For this review, take the finished solid that the model builds, in its own axes (mm). Coordinates: 2 decimals unless noted, no trailing zeros. Write each loop counter-clockwise with the first axis right and the second up, starting at its lowest first coordinate (ties: lowest second). Pieces come first, ordered by that corner, then holes. Notation, with made-up numbers: (-3.5, 55) -> (33.5, 55) arc R9 ccw to (33.5, 66) -> close; hole circle Ø2 at (-8, 22). An arc over 180 degrees is marked (long way). Put each result on its own line as item: value. Start each with the question number.
Item 1: To check wall thickness, follow L1, parallel to X at y = 69.85, z = 4 (3 decimals); L2, parallel to X at y = 59.5, z = 1.5; L3, parallel to X at y = 46, z = 6.25. State the ranges of each line that lie inside material, in increasing order.
Item 2: Consider section B-B on y = 25.4. Give the boundary of the cut face in (x, z), and give its area (3 significant figures).
Item 3: Consider section C-C on z = 1. Give the boundary of the cut face in (x, y) (3 decimals), and give its area (3 significant figures).
Item 4: Consider section A-A on x = 247.65. Give the boundary of the cut face in (y, z), and give its area (3 significant figures).
Item 5: Consider section D-D on y = 50.8. Give the boundary of the cut face in (x, z).
Autodesk Inventor part; units mm, degrees
ref_plane "YZ Plane" through (0, 0, 0) normal (1, 0, 0) x (0, 1, 0)
ref_plane "XZ Plane" through (0, 0, 0) normal (0, 1, 0) x (-1, 0, 0)
ref_plane "XY Plane" through (0, 0, 0) normal (0, 0, 1) x (1, 0, 0)
sketch "Sketch1" plane through (0, 0, 0) normal (0, 0, 1) x (1, 0, 0)
  line L0 (0, 0) -> (444.5, 0)
  line L1 (444.5, 0) -> (444.5, 76.2)
  line L2 (444.5, 76.2) -> (0, 76.2)
  line L3 (0, 76.2) -> (0, 0)
  dimension "d0" = 444.5
  dimension "d1" = 76.2
extrude "Extrusion1" add sketch "Sketch1" along normal blind 6.35
chamfer "Chamfer1" distance 12.7 angle 45 1 edges at (444.5, 0, 3.175)
chamfer "Chamfer2" distance 12.7 angle 45 1 edges at (0, 0, 3.175)
sketch "Sketch2" plane through (0, 0, 6.35) normal (0, 0, 1) x (1, 0, 0)
  line L0 (0, 46.8514) -> (152.4, 46.8514)
  line L1 (444.5, 12.7) -> (444.5, 76.2)
  line L2 (292.1, 46.8514) -> (444.5, 46.8514)
  circle A0 centre (152.4, 46.8514) radius 12.7
  circle A1 centre (292.1, 46.8514) radius 12.7
  point P0 (0, 0)
  point P1 (139.7, 46.8514)
  point P2 (165.1, 46.8514)
  dimension "d10" = 152.4
  dimension "d11" = 25.4
  dimension "d12" = 25.4
extrude "Extrusion2" cut sketch "Sketch2" against normal blind 25.4
sketch "Sketch3" plane through (0, 0, 6.35) normal (0, 0, 1) x (1, 0, 0)
  circle A0 centre (152.4, 46.8514) radius 12.7
  line L0 (139.7, 46.8514) -> (139.7, 76.2)
  line L1 (165.1, 46.8514) -> (165.1, 76.2)
  line L2 (444.5, 76.2) -> (0, 76.2)
  line L3 (139.7, 76.2) -> (165.1, 76.2)
  arc A1 (139.7, 46.8514) -> (165.1, 46.8514) centre (152.4, 46.8514) ccw
  point P0 (0, 0)
extrude "Extrusion3" cut sketch "Sketch3" against normal blind 25.4 contours A0 L0 L2 L1
sketch "Sketch4" plane through (0, 0, 6.35) normal (0, 0, 1) x (1, 0, 0)
  circle A0 centre (292.1, 46.8514) radius 12.7
  line L0 (279.4, 46.8514) -> (279.4, 76.2)
  line L1 (444.5, 76.2) -> (165.1, 76.2)
  line L2 (304.8, 46.8514) -> (304.8, 76.2)
  line L3 (304.8, 76.2) -> (279.4, 76.2)
  arc A1 (279.4, 46.8514) -> (304.8, 46.8514) centre (292.1, 46.8514) ccw
  point P0 (0, 0)
extrude "Extrusion4" cut sketch "Sketch4" against normal blind 25.4 contours A0 L0 L1 L2
sketch "Sketch5" plane through (0, 0, 6.35) normal (0, 0, 1) x (1, 0, 0)
  line L0 (0, 76.2) -> (0, 12.7)
  line L1 (12.7, 0) -> (431.8, 0)
  line L2 (444.5, 12.7) -> (444.5, 76.2)
  circle A0 centre (50.8, 25.4) radius 6.35
  circle A1 centre (393.7, 25.4) radius 6.35
  point P0 (0, 0)
  dimension "d19" = 50.8
  dimension "d20" = 25.4
  dimension "d21" = 25.4
  dimension "d22" = 50.8
  dimension "d23" = 12.7
  dimension "d24" = 12.7
extrude "Extrusion5" cut sketch "Sketch5" against normal blind 25.4
sketch "Sketch6" plane through (0, 0, 6.35) normal (0, 0, 1) x (1, 0, 0)
  line L0 (139.7, 76.2) -> (0, 76.2)
  line L1 (0, 76.2) -> (0, 12.7)
  line L2 (444.5, 76.2) -> (304.8, 76.2)
  line L3 (444.5, 12.7) -> (444.5, 76.2)
  circle A0 centre (6.35, 69.85) radius 0.635
  circle A1 centre (438.15, 69.85) radius 0.635
  point P0 (0, 0)
  dimension "d27" = 6.35
  dimension "d28" = 6.35
  dimension "d29" = 6.35
  dimension "d30" = 6.35
  dimension "d31" = 1.27
  dimension "d32" = 1.27
extrude "Extrusion6" cut sketch "Sketch6" against normal blind 25.4
sketch "Sketch7" plane through (0, 0, 6.35) normal (0, 0, 1) x (1, 0, 0)
  line L0 (279.4, 76.2) -> (165.1, 76.2)
  line L1 (165.1, 76.2) -> (165.1, 46.8514)
  line L2 (279.4, 46.8514) -> (279.4, 76.2)
  circle A0 centre (196.85, 50.8) radius 6.35
  circle A1 centre (247.65, 50.8) radius 6.35
  point P0 (0, 0)
  dimension "d35" = 25.4
  dimension "d36" = 31.75
  dimension "d37" = 25.4
  dimension "d38" = 31.75
  dimension "d39" = 12.7
  dimension "d40" = 12.7
extrude "Extrusion7" cut sketch "Sketch7" against normal blind 25.4
properties part number "Lauren's Part"
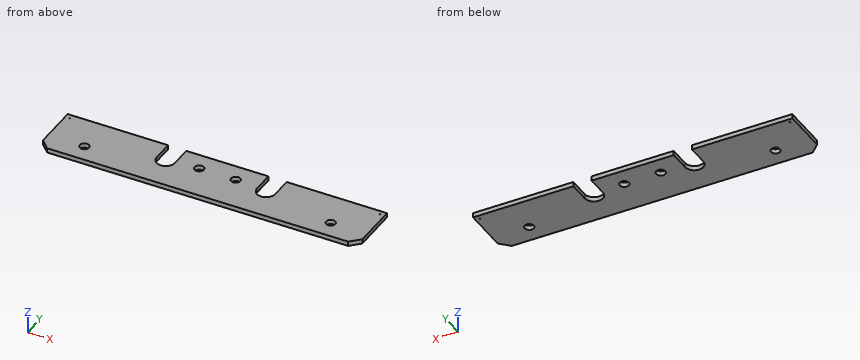
Return value:
1. L1: 0 to 5.715, 6.985 to 139.7, 165.1 to 279.4, 304.8 to 437.515, 438.785 to 444.5
1. L2: 0 to 139.7, 165.1 to 279.4, 304.8 to 444.5
1. L3: 0 to 139.73, 165.07 to 192.69, 201.01 to 243.49, 251.81 to 279.43, 304.77 to 444.5
2. outline: (0, 0) -> (44.45, 0) -> (44.45, 6.35) -> (0, 6.35) -> close; (57.15, 0) -> (387.35, 0) -> (387.35, 6.35) -> (57.15, 6.35) -> close; (400.05, 0) -> (444.5, 0) -> (444.5, 6.35) -> (400.05, 6.35) -> close
2. area: 2,660 mm^2
3. outline: (0, 12.7) -> (12.7, 0) -> (431.8, 0) -> (444.5, 12.7) -> (444.5, 76.2) -> (304.8, 76.2) -> (304.8, 46.851) arc R12.7 cw to (279.4, 46.851) -> (279.4, 76.2) -> (165.1, 76.2) -> (165.1, 46.851) arc R12.7 cw to (139.7, 46.851) -> (139.7, 76.2) -> (0, 76.2) -> close; hole circle Ø1.27 at (6.35, 69.85); hole circle Ø12.7 at (50.8, 25.4); hole circle Ø12.7 at (196.85, 50.8); hole circle Ø12.7 at (247.65, 50.8); hole circle Ø12.7 at (393.7, 25.4); hole circle Ø1.27 at (438.15, 69.85)
3. area: 31,200 mm^2
4. outline: (0, 0) -> (44.45, 0) -> (44.45, 6.35) -> (0, 6.35) -> close; (57.15, 0) -> (76.2, 0) -> (76.2, 6.35) -> (57.15, 6.35) -> close
4. area: 403 mm^2
5. outline: (0, 0) -> (139.7, 0) -> (139.7, 6.35) -> (0, 6.35) -> close; (165.1, 0) -> (190.5, 0) -> (190.5, 6.35) -> (165.1, 6.35) -> close; (203.2, 0) -> (241.3, 0) -> (241.3, 6.35) -> (203.2, 6.35) -> close; (254, 0) -> (279.4, 0) -> (279.4, 6.35) -> (254, 6.35) -> close; (304.8, 0) -> (444.5, 0) -> (444.5, 6.35) -> (304.8, 6.35) -> close
